Model file for the job. Use its own axes, mm. A direction names the side the tool comes from. Give positions to 0.01 mm unless a question says otherwise; leave off trailing zeros. Loops run counter-clockwise (first coordinate to the right, second up) from the corner with the lowest first, then second, coordinate; pieces in that order, holes last. Notation, with made-up numbers: M 26.5,49 L 64.5,49 A27 cw 64.5,74 Z; hole C -18,10 d5. An arc over 180 degrees is marked long. Answer in a Markdown table with one row per item.
```python
from build123d import *

# Parameters (mm, degrees)
SKETCH_1_W          = 53.8
SKETCH_1_H          = 63
EXTRUDE_1_DEPTH     = 3
SKETCH_2_W          = 53.8
SKETCH_2_H          = 1.5
EXTRUDE_2_DEPTH     = 2.8
SKETCH_3_R          = 1
CUT_EXTRUDE_1_DEPTH = 1.5
SKETCH_3_4_R        = 0.7
CUT_EXTRUDE_2_DEPTH = 44.693248906


with BuildPart() as part:
    # 草图1 → 凸台-拉伸1 (new body)
    with BuildSketch(Plane.XY):
        Rectangle(SKETCH_1_W, SKETCH_1_H)
    extrude(amount=EXTRUDE_1_DEPTH)

    # 草图2 → 凸台-拉伸2 (add)
    with BuildSketch(Plane(origin=(0, 31.5, 0), x_dir=(1, 0, 0), z_dir=(0, 1, 0))):
        with Locations((0, -2.25)):
            Rectangle(SKETCH_2_W, SKETCH_2_H)
    extrude(amount=EXTRUDE_2_DEPTH)

    # 草图3 → 切除-拉伸1 (cut)
    with BuildSketch(Plane(origin=(0, 0, 0), x_dir=(-1, 0, 0), z_dir=(0, 0, -1))):
        with Locations((0, -30)):
            Circle(SKETCH_3_R)
    extrude(amount=-CUT_EXTRUDE_1_DEPTH, mode=Mode.SUBTRACT)

    # 草图3<4> → 切除-拉伸2 (cut, through all)
    with BuildSketch(Plane(origin=(0, 0, 0), x_dir=(-1, 0, 0), z_dir=(0, 0, -1))):
        with Locations((0, -30)):
            Circle(SKETCH_3_4_R)
    extrude(amount=-CUT_EXTRUDE_2_DEPTH, mode=Mode.SUBTRACT)


solid = part.part
```
(1) Mould opens along Y. For faces 4 (the flat face through (-26.9, 1, 2)), 5 (the flat face through (0, 34.3, 2)), 6 (the cylindrical face through (0.152, -30.683, 2.24)) say: pulls with the +Y half, pulls with the -Y half, needs draft (parallel to the pull), parting line crosses it, or undercut.
Established:
| item | result |
|---|---|
| face 4 | needs draft |
| face 5 | pulls with the +Y half |
| face 6 | undercut |
(2) Saw through at A-A, the plane y = -30. Give the cut face in (x, z).
Established:
| item | result |
|---|---|
| outline | M -26.9,0 L -1,0 L -1,1.5 L -0.7,1.5 L -0.7,3 L -26.9,3 Z; M 0.7,1.5 L 1,1.5 L 1,0 L 26.9,0 L 26.9,3 L 0.7,3 Z |
(3) Which spindle directions (+Z, -Z, +X, -X, +Y, -Y) get a long thin tool onto all of the face, cutting with end or side? Do faces 1 (the cylindrical face through (0, -29, 1)), 2 (the flat face through (0, 31.5, 1)), 3 (the flat face through (0, -31.5, 1)). Say none if no direction does.
Established:
| item | result |
|---|---|
| face 1 | -Z |
| face 2 | -Z, +X, -X, +Y |
| face 3 | +Z, -Z, +X, -X, -Y |
(4) Saw through at B-B, the plane x = 0. Give the cut face in (y, z).
Established:
| item | result |
|---|---|
| outline | M -31.5,0 L -31,0 L -31,1.5 L -30.7,1.5 L -30.7,3 L -31.5,3 Z; M -29.3,1.5 L -29,1.5 L -29,0 L 31.5,0 L 31.5,1.5 L 34.3,1.5 L 34.3,3 L -29.3,3 Z |
(5) Saw through at C-C, the plane z = 0.65. Give the cut face in (x, y).
Established:
| item | result |
|---|---|
| outline | M -26.9,-31.5 L 26.9,-31.5 L 26.9,31.5 L -26.9,31.5 Z; hole C 0,-30 d2 |
(6) Flat gauge pins, fed straight in: P1, Ø0.8, axis at x = 3, z = 0.5, coming from the +Y side; P2, Ø0.8, axis at x = -10.5, y = 33, coming from the -Z side; P3, Ø1.2, axis at x = 0, y = -30, coming from the +Z side. Where does each tip first touch, or does it go through?
Established:
| item | result |
|---|---|
| P1 | stops at y = 31.5 |
| P2 | stops at z = 1.5 |
| P3 | passes through |
(7) Wall check: L1, parallel to Y at x = 0, z = 0.65; L2, parallel to Y at x = 0, z = 2.6; L3, parallel to Y at x = 23, z = 0.3. Give the ranges that are in metal, low to high.
Established:
| item | result |
|---|---|
| L1 | y = -31.5 to -31, -29 to 31.5 |
| L2 | y = -31.5 to -30.7, -29.3 to 34.3 |
| L3 | y = -31.5 to 31.5 |
